The figure shows three views and two pictorial views of one solid part (mm, origin at its lowest corner). Answer the questions. A direction names the side the tool comes from. Coordinates: 2 decimals unless noted, no trailing zeros. Order: outer loops, then holes, each group sorted by start corner. A loop starts at its lowest first (then second) coordinate and runs counter-clockwise, first axis right, second up.
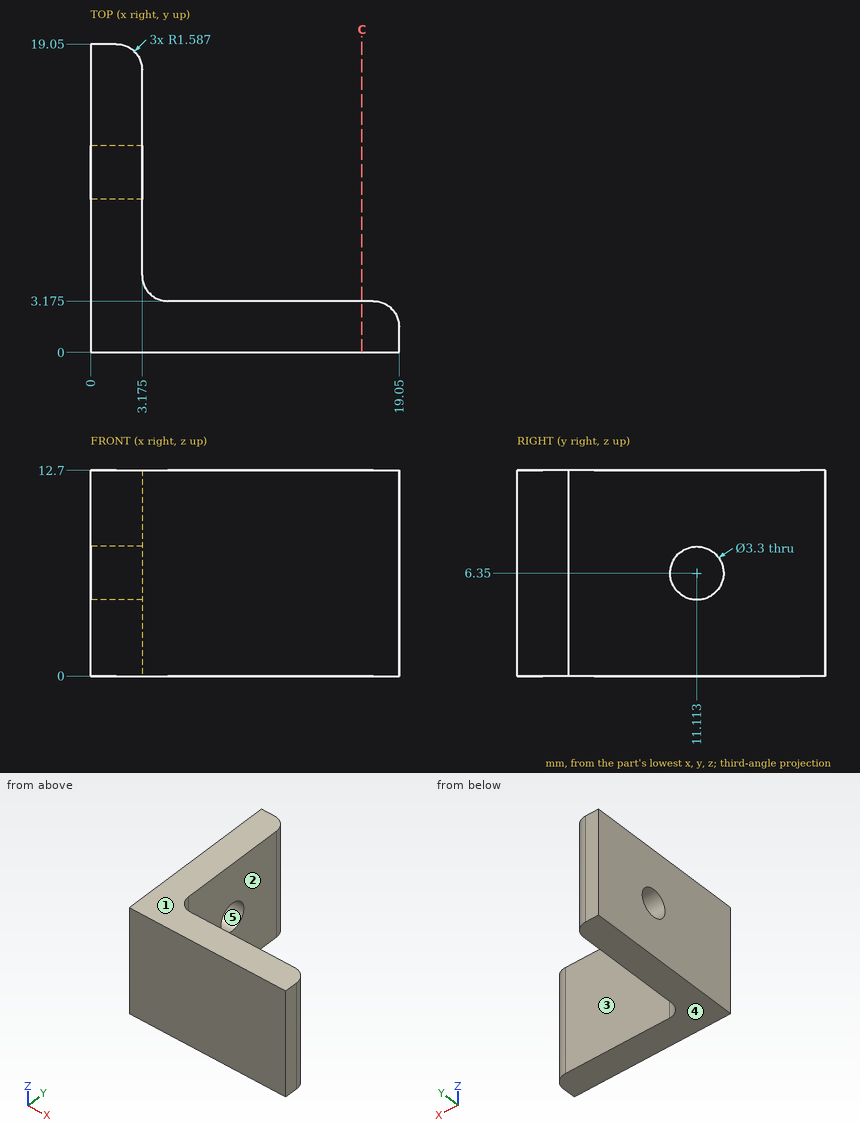
Q1. Which of the six approach directions +Z, -Z, +X, -X, +Y, -Y give full straight-line access (tool end or side, diameter ignored) to the marked faces 1 and 2?
Q2. Determine the mould class of the marked faces 3, 4 and 5 for opening direction Z: +Z half, -Z half, draft (parallel to the pull), parting line (faces both ways), or undercut.
Q3. This flat-tipped pin is pushed along its axis until it touches: P1, Ø3, axis at x = 5, y = 13.5, coming from the -Z side. Where does it stop, or does it pass through?
Q4. The part is cut by section C-C, the plane x = 16.75. Determine the outline of the cut face in (y, z) (1 decimal).
Q5. Straight lines are drawn through the part: L1, parallel to Y at x = 1.4, z = 6.35; L2, parallel to Z at x = 2.25, y = 11; L3, parallel to Y at x = 12.25, z = 10.5 (1 decimal). For each, find the intervals that lie inside material, in ascending order.
Computed values:
1. face 1: +Z, +X, -X, +Y, -Y
1. face 2: +Z, -Z, +X, +Y
2. face 3: draft
2. face 4: -Z half
2. face 5: undercut
3. P1: passes through
4. outline: (0, 0) - (3.2, 0) - (3.2, 12.7) - (0, 12.7) - close
5. L1: y = 0 to 9.46, 12.76 to 19.05
5. L2: z = 0 to 4.7, 8 to 12.7
5. L3: y = 0 to 3.2
